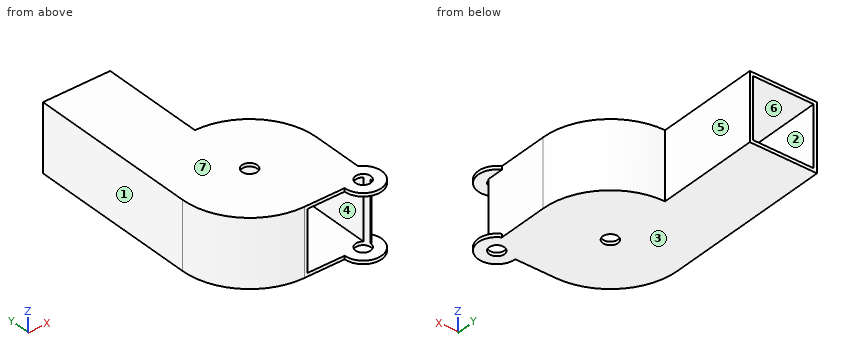
```python
from build123d import *

# Parameters (mm, degrees)
BOSS_EXTRUDE1_DEPTH = 40
SHELL1_T            = -2
SKETCH2_W           = 36
SKETCH2_H           = 36
CUT_EXTRUDE1_DEPTH  = 40
SKETCH7_R           = 11
BOSS_EXTRUDE3_DEPTH = 2
CUT_EXTRUDE4_REACH  = 120.704
SKETCH8_R           = 4.5
BOSS_EXTRUDE4_START = -2
SKETCH9_R           = 11
BOSS_EXTRUDE4_DEPTH = 2
SKETCH10_R          = 4.5
CUT_EXTRUDE5_DEPTH  = 119.70397032


with BuildPart() as part:
    # Sketch1 → Boss-Extrude1 (new body)
    with BuildSketch(Plane.XY):
        with BuildLine():
            Line((-40, 0), (-40, 101.855940277))
            Line((-40, 101.855940277), (0, 101.855940277))
            Line((0, 101.855940277), (0, 40))
            ThreePointArc((0, 40), (28.284271247, 28.284271247), (40, 0))
            Line((40, 0), (40, -40))
            Line((40, -40), (0, -40))
            ThreePointArc((0, -40), (-28.284271247, -28.284271247), (-40, 0))
        make_face()
    extrude(amount=BOSS_EXTRUDE1_DEPTH)

    # Shell1
    shell1_openings = [part.faces().sort_by_distance(p)[0] for p in [
        (-20, 101.855940277, 20),
    ]]
    offset(amount=SHELL1_T, openings=shell1_openings, kind=Kind.INTERSECTION)

    # Sketch2 → Cut-Extrude1 (cut)
    with BuildSketch(Plane.XZ.offset(40)):
        with Locations((20, 20)):
            Rectangle(SKETCH2_W, SKETCH2_H)
    extrude(amount=-CUT_EXTRUDE1_DEPTH, mode=Mode.SUBTRACT)

    # Sketch7 → Boss-Extrude3 (add)
    with BuildSketch(Plane.XY.offset(40)):
        with Locations((35, -40)):
            Circle(SKETCH7_R)
    extrude(amount=-BOSS_EXTRUDE3_DEPTH)

    # Cut-Extrude4: up to this face of the body (flat: up to its plane)
    cut_extrude4_end = Plane(part.part.faces().sort_by_distance((-6.043930541, 21.434186246, 0))[0])
    # Sketch8 → Cut-Extrude4 (cut, up to the picked face)
    with BuildSketch(Plane.XY.offset(40), mode=Mode.PRIVATE) as cut_extrude4_sk1:
        Circle(SKETCH8_R)
    cut_extrude4_tool1 = split(extrude(cut_extrude4_sk1.sketch, amount=-CUT_EXTRUDE4_REACH, mode=Mode.PRIVATE), bisect_by=cut_extrude4_end, keep=Keep.BOTH, mode=Mode.PRIVATE)
    add(cut_extrude4_tool1.solids().sort_by(Axis((0, 0, 40), (0, 0, -1)))[0], mode=Mode.SUBTRACT)

    # Sketch9 → Boss-Extrude4 (add)
    with BuildSketch(Plane(origin=(0, 0, 0), x_dir=(-1, 0, 0), z_dir=(0, 0, -1)).offset(BOSS_EXTRUDE4_START)):
        with Locations((-35, -40)):
            Circle(SKETCH9_R)
    extrude(amount=BOSS_EXTRUDE4_DEPTH)

    # Sketch10 → Cut-Extrude5 (cut, through all)
    with BuildSketch(Plane.XY.offset(40)):
        with Locations((35, -40)):
            Circle(SKETCH10_R)
    extrude(amount=-CUT_EXTRUDE5_DEPTH, mode=Mode.SUBTRACT)


solid = part.part
```
CAD build for the part. Positions are in the model's coordinates, mm. Face numbers are marked on the shaded views. A direction names the side the tool comes from. Coordinates: 2 decimals unless noted, no trailing zeros. Order: outer loops, then holes, each group sorted by start corner. A loop starts at its lowest first (then second) coordinate and runs counter-clockwise, first axis right, second up. Notation, with made-up numbers: (85.5, -39) -> (139.5, -39) arc R25 ccw to (139.5, -15) -> close; hole circle Ø1 at (24.5, 46). An arc over 180 degrees is marked (long way). Use one line per item in the form item = value. Start each with the question number.
1) Band-saw the part on D-D on y = -34. Give the cut face in (x, z), then the cut area to 3 significant figures.
2) Band-saw the part on C-C on x = 35. Give the cut face in (y, z).
3) Pull direction X, two halves, no side cores. Call the marked faces 1, 2 and 3: +X half, -X half, draft (parallel to the pull), parting line (faces both ways), or undercut.
4) Drop flat-ended pins along their axis: pin 1 (12 mm diameter, centred on y = 58, z = 24, fed in from +X); pin 2 (4 mm diameter, centred on y = -20, z = 35.5, fed in from -X); pin 3 (12 mm diameter, centred on y = -17, z = 29.5, fed in from +X). Give the stop position or say it passes through.
5) Drill centre lines: L1, parallel to Z at x = 15, y = -34.5; L2, parallel to X at y = 58, z = 14.5; L3, parallel to X at y = 23, z = 7. Where is each one in solid material? Low to high. Write a range as [from, to].
6) Band-saw the part on B-B on y = 55.5. Give the cut face in (x, z).
7) Tool access for the marked faces 4, 5, 6 and 7: list every direction of +Z, -Z, +X, -X, +Y, -Y with a clear straight run to the whole face (end or side of a thin tool).
8) Band-saw the part on A-A on z = 32. Give the cut face in (x, y).
Entries:
q1.outline = (-21.07, 0) -> (44.22, 0) -> (44.22, 2) -> (40, 2) -> (40, 38) -> (44.22, 38) -> (44.22, 40) -> (-21.07, 40) -> close; hole (-16.97, 2) -> (38, 2) -> (38, 38) -> (-16.97, 38) -> close
q1.area = 481 mm2
q2.outline = (-51, 0) -> (-44.5, 0) -> (-44.5, 2) -> (-51, 2) -> close; (-51, 38) -> (-44.5, 38) -> (-44.5, 40) -> (-51, 40) -> close; (-35.5, 0) -> (19.36, 0) -> (19.36, 40) -> (-35.5, 40) -> (-35.5, 38) -> (14.8, 38) -> (14.8, 2) -> (-35.5, 2) -> close
q3.face_1 = -X half
q3.face_2 = undercut
q3.face_3 = draft
q4.pin_1 = 0
q4.pin_2 = -35.72
q4.pin_3 = 40
q5.L1 = [0, 2], [38, 40]
q5.L2 = [-40, -38], [-2, 0]
q5.L3 = [-40, -38], [30.25, 32.73]
q6.outline = (-40, 0) -> (0, 0) -> (0, 40) -> (-40, 40) -> close; hole (-38, 2) -> (-2, 2) -> (-2, 38) -> (-38, 38) -> close
q7.face_4 = -Y
q7.face_5 = +Z, -Z, +X, +Y
q7.face_6 = none
q7.face_7 = +Z, +X, -X, +Y, -Y
q8.outline = (-40, 0) arc R40 ccw to (0, -40) -> (2, -40) -> (2, -38) -> (0, -38) arc R38 cw to (-38, 0) -> (-38, 101.86) -> (-40, 101.86) -> close; (-2, 37.95) arc R38 cw to (38, 0) -> (38, -36.65) arc R4.5 cw to (39.5, -40) -> (40, -40) -> (40, 0) arc R40 ccw to (0, 40) -> (0, 101.86) -> (-2, 101.86) -> close
